Part model, mm, in its own coordinate system. A direction names the side the tool comes from. Round coordinates to 2 decimals unless told otherwise and drop trailing zeros. Write each loop counter-clockwise with the first axis right and the second up, starting at its lowest first coordinate (ties: lowest second). Pieces come first, ordered by that corner, then holes.
1) Saw through at A-A on z = 1.5. Write the cut outline in (x, y).
2) Drill centre lines: L1, parallel to Y at x = 10, z = 3; L2, parallel to X at y = 22, z = 5; L3, parallel to Y at x = 10, z = 7.5. Where is each one in solid material? Low to high.
3) Saw through at C-C on y = 54. Write the cut outline in (x, z), and give its area (3 significant figures).
4) Saw through at B-B on x = 10. Write the cut outline in (y, z), and give its area (3 significant figures).
5) Pull direction Y, two halves, no side cores. Call faces 1 (the flat face through (10, 5, 6)), 2 (the flat face through (17.1, 4.6, 4.3)), 3 (the cylindrical face through (10.07, 8.75, 3.04)): +Y half, -Y half, draft (parallel to the pull), parting line (faces both ways), or undercut.
6) Which spindle directions (+Z, -Z, +X, -X, +Y, -Y) get a long thin tool onto all of the face, cutting with end or side? Do faces 4 (the flat face through (17, 6, 11)), 5 (the cylindrical face through (9.93, 47.25, 7.6)), 6 (the cylindrical face through (6.18, 6.6, 10.44)). Say none if no direction does.
7) Flat gauge pins, fed straight in: pin 1 (6 mm diameter, centred on x = 13, y = 20, fed in from +Z); pin 2 (1 mm diameter, centred on x = 17.5, z = 5.5, fed in from -Y); pin 3 (2.5 mm diameter, centred on x = 2.5, z = 10.5, fed in from -Y); pin 4 (3.5 mm diameter, centred on x = 9.5, y = 4.5, fed in from +Z). Where does each tip first touch, or does it go through?
8) Saw through at D-D on z = 9.5. Write the cut outline in (x, y), and give its area (3 significant figures).
```python
from build123d import *

# Parameters (mm, degrees)
ESQUISSE1_W             = 20
ESQUISSE1_H             = 60
BOSS_EXTRU_1_DEPTH      = 15
ESQUISSE2_R             = 2.5
ENL_V_MAT_EXTRU_1_DEPTH = 15
ESQUISSE3_W             = 20
ESQUISSE3_H             = 6
ENL_V_MAT_EXTRU_2_DEPTH = 9
ENL_V_MAT_EXTRU_3_DEPTH = 15
ESQUISSE7_W             = 6.5
ESQUISSE7_H             = 8
ENL_V_MAT_EXTRU_4_DEPTH = 9
CONG_1_R                = 2
CHANFREIN1_SIZE         = 3


with BuildPart() as part:
    # Esquisse1 → Boss.-Extru.1 (new body)
    with BuildSketch(Plane.XY):
        with Locations((10, 30)):
            Rectangle(ESQUISSE1_W, ESQUISSE1_H)
    extrude(amount=BOSS_EXTRU_1_DEPTH)

    # Esquisse2 → Enlèv. mat.-Extru.1 (cut)
    with BuildSketch(Plane.XY.offset(15)):
        with Locations((10, 54)):
            Circle(ESQUISSE2_R)
        with BuildLine():
            Line((6.75, 12), (6.75, 44))
            ThreePointArc((6.75, 44), (10, 47.25), (13.25, 44))
            Line((13.25, 44), (13.25, 12))
            ThreePointArc((13.25, 12), (10, 8.75), (6.75, 12))
        make_face()
    extrude(amount=-ENL_V_MAT_EXTRU_1_DEPTH, mode=Mode.SUBTRACT)

    # Esquisse3 → Enlèv. mat.-Extru.2 (cut)
    with BuildSketch(Plane.XY.offset(15)):
        with Locations((10, 3)):
            Rectangle(ESQUISSE3_W, ESQUISSE3_H)
    extrude(amount=-ENL_V_MAT_EXTRU_2_DEPTH, mode=Mode.SUBTRACT)

    # Esquisse6 → Enlèv. mat.-Extru.3 (cut)
    with BuildSketch(Plane.XY.offset(15)):
        Polygon((7.5, 0), (0, 7.5), (0, -7.5), (20, -7.5), (20, 7.5), (12.5, 0), align=None)
    extrude(amount=-ENL_V_MAT_EXTRU_3_DEPTH, mode=Mode.SUBTRACT)

    # Esquisse7 → Enlèv. mat.-Extru.4 (cut)
    with BuildSketch(Plane.XY.offset(15)):
        with Locations((10, 10)):
            Rectangle(ESQUISSE7_W, ESQUISSE7_H)
    extrude(amount=-ENL_V_MAT_EXTRU_4_DEPTH, mode=Mode.SUBTRACT)

    # Congé1
    cong_1_edges = [part.edges().sort_by_distance(p)[0] for p in [
        (6.75, 6, 10.5),
        (13.25, 6, 10.5),
    ]]
    fillet(cong_1_edges, radius=CONG_1_R)

    # Chanfrein1
    chanfrein1_edges = [part.edges().sort_by_distance(p)[0] for p in [
        (0, 60, 7.5),
        (20, 60, 7.5),
    ]]
    chamfer(chanfrein1_edges, length=CHANFREIN1_SIZE)


solid = part.part
```
Completed:
1. outline: (0, 7.5) - (7.5, 0) - (12.5, 0) - (20, 7.5) - (20, 57) - (17, 60) - (3, 60) - (0, 57) - close; hole (6.75, 12) arc R3.25 ccw to (13.25, 12) - (13.25, 44) arc R3.25 ccw to (6.75, 44) - close; hole circle Ø5 at (10, 54)
2. L1: y = 0 to 8.75, 47.25 to 51.5, 56.5 to 60
2. L2: x = 0 to 6.75, 13.25 to 20
2. L3: y = 47.25 to 51.5, 56.5 to 60
3. outline: (0, 0) - (7.5, 0) - (7.5, 15) - (0, 15) - close; (12.5, 0) - (20, 0) - (20, 15) - (12.5, 15) - close
3. area: 225 mm2
4. outline: (0, 0) - (8.75, 0) - (8.75, 6) - (0, 6) - close; (47.25, 0) - (51.5, 0) - (51.5, 15) - (47.25, 15) - close; (56.5, 0) - (60, 0) - (60, 15) - (56.5, 15) - close
4. area: 169 mm2
5. face 1: draft
5. face 2: -Y half
5. face 3: undercut
6. face 4: +Z, +X, -X, -Y
6. face 5: +Z, -Z
6. face 6: +Z, -Y
7. pin 1: stops at z = 15
7. pin 2: stops at y = 4.5
7. pin 3: stops at y = 6
7. pin 4: stops at z = 6
8. outline: (0, 7.5) - (1.5, 6) - (4.75, 6) arc R2 ccw to (6.75, 8) - (6.75, 44) arc R3.25 cw to (13.25, 44) - (13.25, 8) arc R2 ccw to (15.25, 6) - (18.5, 6) - (20, 7.5) - (20, 57) - (17, 60) - (3, 60) - (0, 57) - close; hole circle Ø5 at (10, 54)
8. area: 784 mm2
